Design review of the part shown in the three views and the two pictorial views. Dimensions are in mm from the part's minimum x, y and z. Give positions to 0.01 mm unless a question says otherwise; leave off trailing zeros. Order: outer loops, then holes, each group sorted by start corner. A loop starts at its lowest first (then second) coordinate and runs counter-clockwise, first axis right, second up. Notation, with made-up numbers: (-37.75, 74) -> (-33.75, 74) arc R29 cw to (-33.75, 101) -> close; hole circle Ø4 at (-3, 80.5). An arc over 180 degrees is marked (long way). Answer in a Markdown table with one row per item. Add a question column.
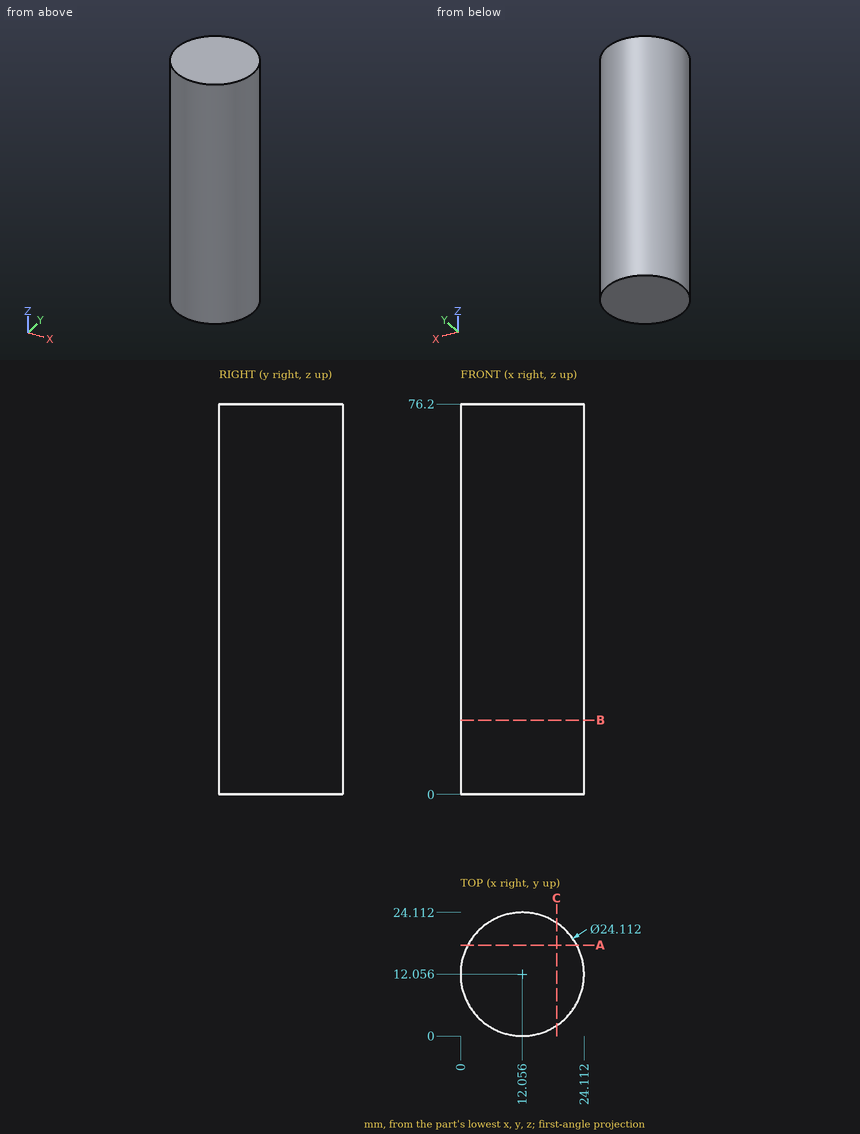
1) Add section C-C, the plane x = 18.75. Write out the cut boundary in (y, z).
2) Clearance check with flat-ended pins moving along their axes: P1, Ø2, axis at y = 18, z = 31, coming from the +X side; P2, Ø3, axis at x = 14, z = 21, coming from the +Y side; P3, Ø1.5, axis at x = 18, z = 43.5, coming from the -Y side; P4, Ø12, axis at y = 8.5, z = 54, coming from the +X side. State where each tip first meets the part, or that it passes through.
3) For L1, parallel to X at y = 19, z = 20; L2, parallel to Y at x = 17.5, z = 47.5; L3, parallel to X at y = 17.25, z = 23, list the stretches that pass through material, from the lowest coordinate up.
4) Add section A-A, the plane y = 17.75. Write out the cut boundary in (x, z).
5) Add section B-B, the plane z = 14.5. Write out the cut boundary in (x, y).
Verdict:
| question | item | result |
|---|---|---|
| 1 | outline | (2.03, 0) -> (22.08, 0) -> (22.08, 76.2) -> (2.03, 76.2) -> close |
| 2 | P1 | stops at x = 23.05 |
| 2 | P2 | stops at y = 24.1 |
| 2 | P3 | stops at y = 1.18 |
| 2 | P4 | stops at x = 24.11 |
| 3 | L1 | x = 2.2 to 21.91 |
| 3 | L2 | y = 1.3 to 22.81 |
| 3 | L3 | x = 1.18 to 22.94 |
| 4 | outline | (1.43, 0) -> (22.68, 0) -> (22.68, 76.2) -> (1.43, 76.2) -> close |
| 5 | outline | circle Ø24.11 at (12.06, 12.06) |
